from build123d import *

# Parameters (mm, degrees)
SKETCH1_W           = 150
SKETCH1_H           = 150
BOSS_EXTRUDE1_DEPTH = 3
CUT_EXTRUDE1_DEPTH  = 264.0332057
SKETCH4_R           = 2.5
CUT_EXTRUDE2_DEPTH  = 3
SKETCH5_W           = 156
SKETCH5_H           = 156
SKETCH5_W_2         = 150
SKETCH5_H_2         = 150
BOSS_EXTRUDE2_DEPTH = 3
SKETCH6_R           = 2
CUT_EXTRUDE3_DEPTH  = 10


with BuildPart() as part:
    # Sketch1 → Boss-Extrude1 (new body)
    with BuildSketch(Plane.XY):
        with Locations((146.896551724, 66.206896552)):
            Rectangle(SKETCH1_W, SKETCH1_H)
    extrude(amount=BOSS_EXTRUDE1_DEPTH)

    # Sketch2 → Cut-Extrude1 (cut, through all)
    with BuildSketch(Plane.XY.offset(3)):
        with BuildLine():
            ThreePointArc((188.163122783, 113.13032186), (146.896551724, 128.694797217), (105.629980666, 113.13032186))
            Line((105.629980666, 113.13032186), (112.718359737, 106.041942789))
            ThreePointArc((112.718359737, 106.041942789), (146.896551724, 118.694797217), (181.074743712, 106.041942789))
            Line((181.074743712, 106.041942789), (188.163122783, 113.13032186))
        make_face()
        with BuildLine():
            Line((107.061505487, 100.385088539), (99.973126416, 107.47346761))
            ThreePointArc((99.973126416, 107.47346761), (84.408651059, 66.206896552), (99.973126416, 24.940325493))
            Line((99.973126416, 24.940325493), (107.061505487, 32.028704564))
            ThreePointArc((107.061505487, 32.028704564), (94.408651059, 66.206896552), (107.061505487, 100.385088539))
        make_face()
        with BuildLine():
            ThreePointArc((209.384452389, 66.206896552), (205.363995952, 88.259009716), (193.819977032, 107.47346761))
            Line((193.819977032, 107.47346761), (186.731597961, 100.385088539))
            ThreePointArc((186.731597961, 100.385088539), (196.119705149, 84.429434333), (199.384452389, 66.206896552))
            ThreePointArc((199.384452389, 66.206896552), (196.119705149, 47.984358771), (186.731597961, 32.028704564))
            Line((186.731597961, 32.028704564), (193.819977032, 24.940325493))
            ThreePointArc((193.819977032, 24.940325493), (205.363995952, 44.154783387), (209.384452389, 66.206896552))
        make_face()
        with BuildLine():
            Line((112.718359737, 26.371850315), (105.629980666, 19.283471244))
            ThreePointArc((105.629980666, 19.283471244), (146.896551724, 3.718995886), (188.163122783, 19.283471244))
            Line((188.163122783, 19.283471244), (181.074743712, 26.371850315))
            ThreePointArc((181.074743712, 26.371850315), (146.896551724, 13.718995886), (112.718359737, 26.371850315))
        make_face()
        with BuildLine():
            ThreePointArc((150.896551724, 23.907703853), (176.940034403, 36.163413873), (189.195744423, 62.206896552))
            Line((189.195744423, 62.206896552), (179.137266506, 62.206896552))
            ThreePointArc((179.137266506, 62.206896552), (169.868966591, 43.234481685), (150.896551724, 33.96618177))
            Line((150.896551724, 33.96618177), (150.896551724, 23.907703853))
        make_face()
        with BuildLine():
            Line((114.655836942, 62.206896552), (104.597359026, 62.206896552))
            ThreePointArc((104.597359026, 62.206896552), (116.853069045, 36.163413873), (142.896551724, 23.907703853))
            Line((142.896551724, 23.907703853), (142.896551724, 33.96618177))
            ThreePointArc((142.896551724, 33.96618177), (123.924136857, 43.234481685), (114.655836942, 62.206896552))
        make_face()
        with BuildLine():
            Line((142.896551724, 98.447611333), (142.896551724, 108.50608925))
            ThreePointArc((142.896551724, 108.50608925), (116.853069045, 96.250379231), (104.597359026, 70.206896552))
            Line((104.597359026, 70.206896552), (114.655836942, 70.206896552))
            ThreePointArc((114.655836942, 70.206896552), (123.924136857, 89.179311419), (142.896551724, 98.447611333))
        make_face()
        with BuildLine():
            ThreePointArc((189.195744423, 70.206896552), (176.940034403, 96.250379231), (150.896551724, 108.50608925))
            Line((150.896551724, 108.50608925), (150.896551724, 98.447611333))
            ThreePointArc((150.896551724, 98.447611333), (169.868966591, 89.179311419), (179.137266506, 70.206896552))
            Line((179.137266506, 70.206896552), (189.195744423, 70.206896552))
        make_face()
        with BuildLine():
            Line((165.372753073, 79.026243651), (158.090015102, 71.74350568))
            ThreePointArc((158.090015102, 71.74350568), (159.056537781, 69.049853135), (159.384452389, 66.206896552))
            ThreePointArc((159.384452389, 66.206896552), (159.166880972, 63.885973637), (158.521748029, 61.645923641))
            Line((158.521748029, 61.645923641), (165.932760465, 54.234911206))
            ThreePointArc((165.932760465, 54.234911206), (168.504305512, 59.977076926), (169.384452389, 66.206896552))
            ThreePointArc((169.384452389, 66.206896552), (168.358106385, 72.923096956), (165.372753073, 79.026243651))
        make_face()
        with BuildLine():
            Line((134.077204625, 84.6830979), (141.359942596, 77.400359929))
            ThreePointArc((141.359942596, 77.400359929), (146.896551724, 78.694797217), (152.433160852, 77.400359929))
            Line((152.433160852, 77.400359929), (159.715898823, 84.6830979))
            ThreePointArc((159.715898823, 84.6830979), (146.896551724, 88.694797217), (134.077204625, 84.6830979))
        make_face()
        with BuildLine():
            ThreePointArc((135.703088346, 60.670287424), (134.408651059, 66.206896552), (135.703088346, 71.74350568))
            Line((135.703088346, 71.74350568), (128.420350375, 79.026243651))
            ThreePointArc((128.420350375, 79.026243651), (124.408651059, 66.206896552), (128.420350375, 53.387549452))
            Line((128.420350375, 53.387549452), (135.703088346, 60.670287424))
        make_face()
        with BuildLine():
            ThreePointArc((152.433160852, 55.013433174), (146.896551724, 53.718995886), (141.359942596, 55.013433174))
            Line((141.359942596, 55.013433174), (134.077204625, 47.730695203))
            ThreePointArc((134.077204625, 47.730695203), (146.896551724, 43.718995886), (159.715898823, 47.730695203))
            Line((159.715898823, 47.730695203), (152.433160852, 55.013433174))
        make_face()
    extrude(amount=-CUT_EXTRUDE1_DEPTH, mode=Mode.SUBTRACT)

    # Sketch4 → Cut-Extrude2 (cut)
    with BuildSketch(Plane.XY.offset(3)):
        with Locations((81.896551724, 131.206896552)):
            Circle(SKETCH4_R)
        with Locations((211.896551724, 131.206896552)):
            Circle(SKETCH4_R)
        with Locations((211.896551724, 1.206896552)):
            Circle(SKETCH4_R)
        with Locations((81.896551724, 1.206896552)):
            Circle(SKETCH4_R)
    extrude(amount=-CUT_EXTRUDE2_DEPTH, mode=Mode.SUBTRACT)

    # Sketch5 → Boss-Extrude2 (add)
    with BuildSketch(Plane(origin=(0, 0, 0), x_dir=(-1, 0, 0), z_dir=(0, 0, -1))):
        with Locations((-146.896551724, 66.206896552)):
            Rectangle(SKETCH5_W, SKETCH5_H)
        with Locations((-146.896551724, 66.206896552)):
            Rectangle(SKETCH5_W_2, SKETCH5_H_2, mode=Mode.SUBTRACT)
    extrude(amount=-BOSS_EXTRUDE2_DEPTH)

    # Sketch6 → Cut-Extrude3 (cut)
    with BuildSketch(Plane.XY.offset(3)):
        with Locations((146.896551724, 66.206896552)):
            Circle(SKETCH6_R)
    extrude(amount=-CUT_EXTRUDE3_DEPTH, mode=Mode.SUBTRACT)


solid = part.part
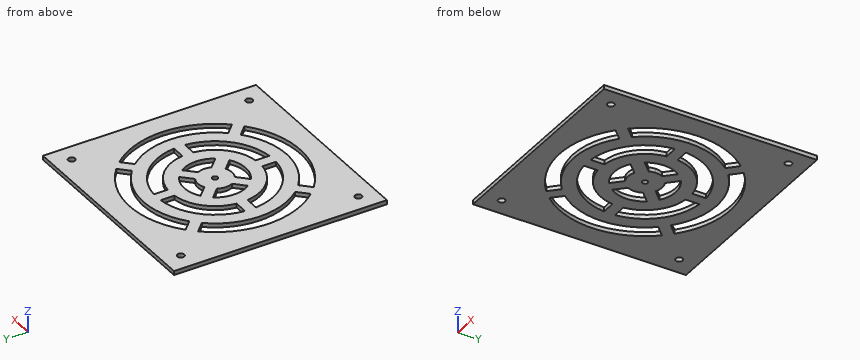
Work out the finished part from the listing and answer in its coordinate system (mm). Give positions to 0.01 mm unless a question says otherwise; leave off trailing zeros. Write each loop counter-clockwise with the first axis right and the second up, starting at its lowest first coordinate (ties: lowest second). Pieces come first, ordered by that corner, then holes. Notation, with made-up numbers: (3, 35) - (32, 35) arc R27 ccw to (32, 72) - close; hole circle Ø8 at (43, 9). An arc over 180 degrees is marked (long way). One line per item, written item: value. Start each with the question number.
1. Consider probe 1 along X at (y, z) = (66, 1.6); probe 2 along Y at (x, z) = (114, 1.15); probe 3 along X at (y, z) = (3.5, 2.2). Determine where each line is inside the solid, lowest interval first.
2. Find section D-D (y = 9.5). Write down the section's boundary in (x, z), then the cut area to 4 significant figures.
3. Find section B-B (y = 90.5). Write down the section's boundary in (x, z), then the cut area to 3 significant figures.
4. Find section C-C (x = 155). Write down the section's boundary in (y, z).
5. Find section A-A (x = 130.5). Write down the section's boundary in (y, z), then the cut area to 3 significant figures.
Geometry results:
1. probe 1: 68.9 to 84.41, 94.41 to 124.41, 134.41 to 144.91, 148.89 to 159.38, 169.38 to 199.38, 209.38 to 224.9
1. probe 2: -11.79 to 13.08, 25.31 to 39.32, 62.21 to 70.21, 93.1 to 107.11, 119.33 to 144.21
1. probe 3: 68.9 to 80.9, 82.89 to 210.9, 212.89 to 224.9
2. outline: (68.9, 0) - (120.65, 0) - (120.65, 3) - (68.9, 3) - close; (173.15, 0) - (224.9, 0) - (224.9, 3) - (173.15, 3) - close
2. area: 310.5 mm2
3. outline: (68.9, 0) - (89.32, 0) - (89.32, 3) - (68.9, 3) - close; (100.37, 0) - (112.04, 0) - (112.04, 3) - (100.37, 3) - close; (125.33, 0) - (168.47, 0) - (168.47, 3) - (125.33, 3) - close; (181.75, 0) - (193.42, 0) - (193.42, 3) - (181.75, 3) - close; (204.47, 0) - (224.9, 0) - (224.9, 3) - (204.47, 3) - close
3. area: 322 mm2
4. outline: (-11.79, 0) - (4.25, 0) - (4.25, 3) - (-11.79, 3) - close; (14.35, 0) - (24.5, 0) - (24.5, 3) - (14.35, 3) - close; (34.75, 0) - (45.23, 0) - (45.23, 3) - (34.75, 3) - close; (52.45, 0) - (79.97, 0) - (79.97, 3) - (52.45, 3) - close; (87.18, 0) - (97.67, 0) - (97.67, 3) - (87.18, 3) - close; (107.91, 0) - (118.07, 0) - (118.07, 3) - (107.91, 3) - close; (128.17, 0) - (144.21, 0) - (144.21, 3) - (128.17, 3) - close
5. outline: (-11.79, 0) - (5.91, 0) - (5.91, 3) - (-11.79, 3) - close; (16.35, 0) - (27.01, 0) - (27.01, 3) - (16.35, 3) - close; (38.16, 0) - (55.47, 0) - (55.47, 3) - (38.16, 3) - close; (76.95, 0) - (94.25, 0) - (94.25, 3) - (76.95, 3) - close; (105.4, 0) - (116.07, 0) - (116.07, 3) - (105.4, 3) - close; (126.51, 0) - (144.21, 0) - (144.21, 3) - (126.51, 3) - close
5. area: 274 mm2
